Design review of the part built by this model. Coordinates are the model's own, in mm. Face numbers are marked on the shaded views. A direction names the side the tool comes from. Round coordinates to 2 decimals unless told otherwise and drop trailing zeros. Write each loop counter-clockwise with the first axis right and the second up, starting at its lowest first coordinate (ties: lowest second). Pieces come first, ordered by that corner, then holes. Notation, with made-up numbers: M 45,53 L 94,53 A17 cw 94,60 Z; hole C 69.25,23.5 d10. An arc over 180 degrees is marked long. One line per question, with ' | ' between items. Start each with the question number.
Item 1: Draft analysis for pull direction Y (two halves, no side actions). For the marked faces 3, 4, 5 and 6, state which applies: released by +Y, released by -Y, zero draft, split by the parting line, or undercut.
Item 2: Add section B-B, the plane x = 15. State the section outline as (y, z) points, and give its area (3 significant figures).
Item 3: Machinability: for the marked faces 1 and 2, which of the approach directions +Z, -Z, +X, -X, +Y, -Y give a long, thin tool a straight path to every point of the face, cutting with its end or side? Answer none if there is none.
Item 4: Insertion check: pin 1 Ø3 at (y, z) = (-20, -140) entering from +X; pin 2 Ø9 at (x, y) = (16, -91) entering from -Z; pin 3 Ø3 at (y, z) = (-80, -141.5) entering from -X; pin 4 Ø2 at (y, z) = (-45, -91.5) entering from +X. Each pin has a flat end and moves straight along its axis. Give the tip position at first contact, or say it passes through.
Item 5: Add section C-C, the plane x = 25.5. State the section outline as (y, z) points.
Item 6: Add section D-D, the plane y = -45. State the section outline as (x, z) points.
Item 7: For L1, parallel to Z at x = -4.45, y = -140; L2, parallel to Y at x = -7.6, z = -140; L3, parallel to Y at x = -5, z = -8.5, list the stretches that pass through material, from the lowest coordinate up.
Item 8: Add section A-A, the plane y = -80. State the section outline as (x, z) points.
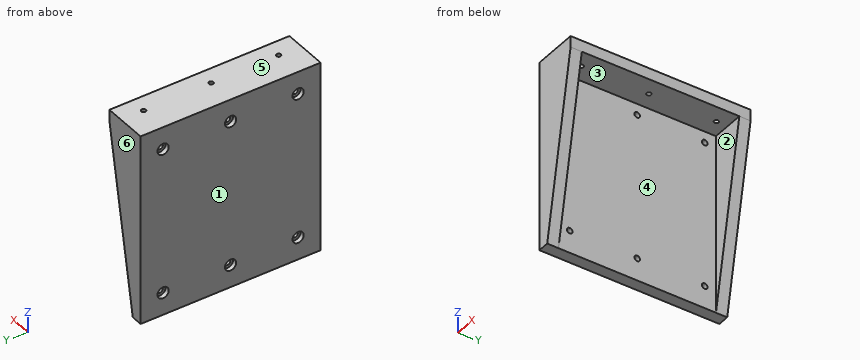
Autodesk Inventor part; units mm, degrees
ref_plane "YZ Plane" through (0, 0, 0) normal (1, 0, 0) x (0, 1, 0)
ref_plane "XZ Plane" through (0, 0, 0) normal (0, 1, 0) x (-1, 0, 0)
ref_plane "XY Plane" through (0, 0, 0) normal (0, 0, 1) x (1, 0, 0)
sketch "Sketch21" plane through (0, 0, 0) normal (0, 0, 1) x (1, 0, 0)
  line L0 (0, 0) -> (30, 0)
  line L1 (30, 0) -> (30, -160)
  line L2 (30, -160) -> (0, -160)
  line L3 (0, -160) -> (0, 0)
  dimension "d53" = 30
  dimension "d1" = 160
extrude "Extrusion15" add sketch "Sketch21" along normal blind 10
sketch "Sketch22" plane through (0, -160, 0) normal (-1, 0, 0) x (0, 0, 1)
  line L0 (0, 160) -> (10, 160)
  line L1 (10, 160) -> (-160, 160)
  line L2 (-160, 160) -> (-160, 0)
  line L3 (-160, 0) -> (10, 0)
  line L4 (10, 0) -> (10, 160)
  dimension "d57" = 170
  dimension "d58" = 160
extrude "Extrusion16" add sketch "Sketch22" along normal blind 10
sketch "Sketch23" plane through (30, 0, 10) normal (0, 1, 0) x (1, 0, 0)
  line L0 (-30, 170) -> (-40, 170)
  line L1 (0, 10) -> (0, 0)
  line L2 (-30, 170) -> (0, 10)
  line L3 (-30, 10) -> (0, 10)
  line L4 (0, 10) -> (-30, 10)
  line L5 (-30, 10) -> (-30, 170)
  line L6 (-40, 170) -> (-40, 0)
extrude "Extrusion17" add sketch "Sketch23" against normal blind 10
sketch "Sketch24" plane through (30, -160, 0) normal (0, -1, 0) x (1, 0, 0)
  line L0 (-30, -160) -> (-40, -160)
  line L1 (-30, 0) -> (0, 0)
  line L2 (-30, -160) -> (-30, 0)
  line L3 (0, 0) -> (0, 10)
  line L4 (-30, 0) -> (0, 0)
  line L5 (-30, -160) -> (0, 0)
  line L6 (0, 0) -> (-30, -160)
extrude "Extrusion18" add sketch "Sketch24" against normal blind 10
sketch "Sketch25" plane through (0, 0, 10) normal (0, 0, 1) x (1, 0, 0)
  circle A0 centre (15, -20) radius 2
  circle A1 centre (15, -80) radius 2
  circle A2 centre (15, -140) radius 2
  line L0 (30, -160) -> (-10, -160)
  line L1 (30, 0) -> (-10, 0)
  point P0 (0, 0)
  dimension "d65" = 4
  dimension "d66" = 4
  dimension "d67" = 4
  dimension "d70" = 20
  dimension "d71" = 20
  dimension "d72" = 80
extrude "Extrusion19" cut sketch "Sketch25" against normal blind 20
sketch "Sketch27" plane through (-10, -160, 0) normal (-1, 0, 0) x (0, 0, 1)
  circle A0 centre (-10, 20) radius 2.5
  line L0 (-160, 0) -> (10, 0)
  circle A1 centre (-10, 80) radius 2.5
  circle A2 centre (-10, 140) radius 2.5
  line L1 (10, 160) -> (-160, 160)
  line L2 (10, 0) -> (10, 160)
  circle A3 centre (-140, 80) radius 2.5
  line L3 (-160, 160) -> (-160, 0)
  circle A4 centre (-140, 20) radius 2.5
  circle A5 centre (-140, 140) radius 2.5
  point P0 (0, 160)
  dimension "d73" = 20
  dimension "d74" = 5
  dimension "d75" = 5
  dimension "d76" = 80
  dimension "d77" = 5
  dimension "d78" = 20
  dimension "d79" = 20
  dimension "d80" = 20
  dimension "d81" = 20
  dimension "d84" = 5
  dimension "d85" = 20
  dimension "d86" = 80
  dimension "d87" = 5
  dimension "d88" = 20
  dimension "d89" = 20
  dimension "d90" = 5
  dimension "d91" = 20
  dimension "d92" = 20
extrude "Extrusion20" cut sketch "Sketch27" against normal blind 20 contours A0 | A1 | A2 | A3 | A4 | A5
sketch "Sketch29" plane through (-10, -160, 0) normal (-1, 0, 0) x (0, 0, 1)
  circle A0 centre (-140, 80) radius 2.5
  circle A1 centre (-140, 80) radius 5
  circle A2 centre (-140, 20) radius 2.5
  circle A3 centre (-140, 20) radius 5
  circle A4 centre (-140, 140) radius 2.5
  circle A5 centre (-140, 140) radius 5
  circle A6 centre (-10, 20) radius 2.5
  circle A7 centre (-10, 20) radius 5
  circle A8 centre (-10, 80) radius 2.5
  circle A9 centre (-10, 80) radius 5
  circle A10 centre (-10, 140) radius 2.5
  circle A11 centre (-10, 140) radius 5
  point P0 (0, 160)
  dimension "d93" = 10
  dimension "d94" = 10
  dimension "d95" = 10
  dimension "d96" = 10
  dimension "d97" = 10
  dimension "d98" = 10
extrude "Extrusion21" cut sketch "Sketch29" against normal blind 4 contours A0 | A1 | A2 | A3 | A4 | A5 | A6 | A7 | A8 | A9 | A10 | A11
equation "\"d58\" = d1"
equation "\"d65\" = d67"
equation "\"d66\" = d67"
equation "\"d71\" = d70"
equation "\"d73\" = d70"
equation "\"d74\" = d75"
equation "\"d76\" = d72"
equation "\"d77\" = d75"
equation "\"d78\" = d70"
equation "\"d80\" = d79"
equation "\"d81\" = d79"
equation "\"d84\" = d75"
equation "\"d85\" = d79"
equation "\"d86\" = d72"
equation "\"d87\" = d75"
equation "\"d88\" = d79"
equation "\"d89\" = d70"
equation "\"d90\" = d75"
equation "\"d91\" = d79"
equation "\"d92\" = d70"
equation "\"d94\" = d93"
equation "\"d95\" = d93"
equation "\"d96\" = d93"
equation "\"d97\" = d93"
equation "\"d98\" = d93"
properties part number "bracket_v02"
Computed values:
1) face 3: undercut | face 4: undercut | face 5: zero draft | face 6: released by +Y
2) outline: M -160,-80 L -150,-80 L -150,0 L -142,0 L -142,10 L -160,10 Z; M -138,0 L -82,0 L -82,10 L -138,10 Z; M -78,0 L -22,0 L -22,10 L -78,10 Z; M -18,0 L -10,0 L -10,-80 L 0,-80 L 0,10 L -18,10 Z | area: 3,080 mm^2
3) face 1: +Z, -Z, -X, +Y, -Y | face 2: -Z, +X
4) pin 1: passes through | pin 2: stops at z = 0 | pin 3: stops at x = -6 | pin 4: stops at x = 0
5) outline: M -160,-24 L -150,-24 L -150,0 L -10,0 L -10,-24 L 0,-24 L 0,10 L -160,10 Z
6) outline: M -10,-160 L 0,-160 L 0,0 L 30,0 L 30,10 L -10,10 Z
7) L1: z = -160 to -142.5, -137.5 to -12.5, -7.5 to 10 | L2: y = -160 to -145, -135 to -85, -75 to -25, -15 to 0 | L3: y = -160 to -142, -138 to -82, -78 to -22, -18 to 0
8) outline: M -10,-160 L 0,-160 L 0,-142.5 L -6,-142.5 L -6,-145 L -10,-145 Z; M -10,-135 L -6,-135 L -6,-137.5 L 0,-137.5 L 0,-12.5 L -6,-12.5 L -6,-15 L -10,-15 Z; M -10,-5 L -6,-5 L -6,-7.5 L 0,-7.5 L 0,0 L 13,0 L 13,10 L -10,10 Z; M 17,0 L 30,0 L 30,10 L 17,10 Z
